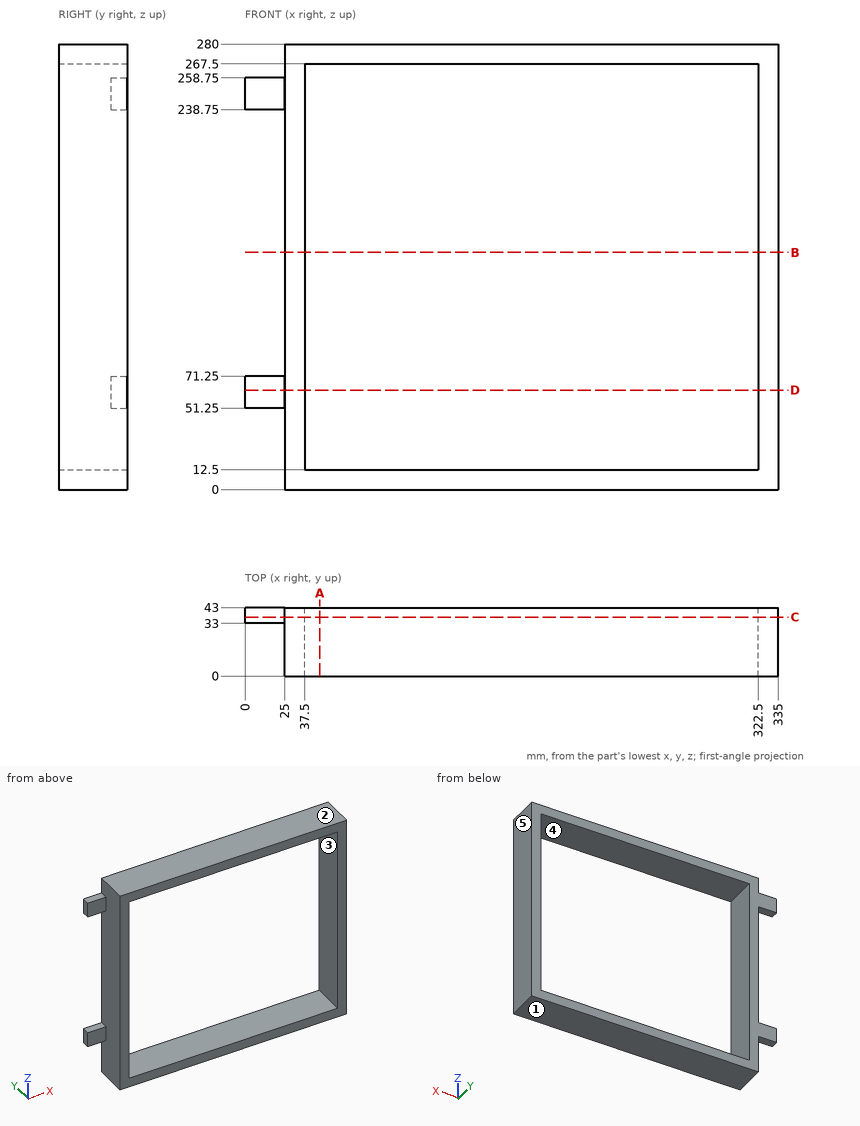
Here's the drawing with two shaded views (mm, measured from the low corner). I have some questions. A direction names the side the tool comes from. Round coordinates to 2 decimals unless told otherwise and drop trailing zeros. Order: outer loops, then holes, each group sorted by start corner. A loop starts at its lowest first (then second) coordinate and runs counter-clockwise, first axis right, second up. Notation, with made-up numbers: M 55,55.25 L 100,55.25 A14 ccw 100,76.25 Z; hole C 1.25,84.5 d3. An arc over 180 degrees is marked long. Answer in a Markdown table with one row per item.
Item 1: Imagine slicing it at C-C, the plane y = 37. Write out the boundary of the cut face in (x, z).
A:
| item | result |
|---|---|
| outline | M 0,51.25 L 25,51.25 L 25,0 L 335,0 L 335,280 L 25,280 L 25,258.75 L 0,258.75 L 0,238.75 L 25,238.75 L 25,71.25 L 0,71.25 Z; hole M 37.5,12.5 L 322.5,12.5 L 322.5,267.5 L 37.5,267.5 Z |
Item 2: Imagine slicing it at A-A, the plane x = 47. Write out the boundary of the cut face in (y, z).
A:
| item | result |
|---|---|
| outline | M 0,0 L 43,0 L 43,12.5 L 0,12.5 Z; M 0,267.5 L 43,267.5 L 43,280 L 0,280 Z |
Item 3: If I drill on L1, parallel to Z at x = 251.5, y = 13; L2, parallel to X at y = 40, z = 257; L3, parallel to X at y = 13, z = 101, over which ranges is the centre line in solid material (lowest first)? Write a range as from..to.
A:
| item | result |
|---|---|
| L1 | z = 0..12.5, 267.5..280 |
| L2 | x = 0..37.5, 322.5..335 |
| L3 | x = 25..37.5, 322.5..335 |
Item 4: Imagine slicing it at D-D, the plane z = 62.5. Write out the boundary of the cut face in (x, y), and give its area (4 significant figures).
A:
| item | result |
|---|---|
| outline | M 0,33 L 25,33 L 25,0 L 37.5,0 L 37.5,43 L 0,43 Z; M 322.5,0 L 335,0 L 335,43 L 322.5,43 Z |
| area | 1,325 mm2 |
Item 5: I'm going to push flat-ended pins straight in: pin 1 (8 mm diameter, centred on x = 15.5, y = 37, fed in from -Z); pin 2 (5 mm diameter, centred on x = 7, y = 39, fed in from +Z); pin 3 (21.5 mm diameter, centred on y = 29.5, z = 101.5, fed in from -X). Where does each tip first touch, or does it pass through?
A:
| item | result |
|---|---|
| pin 1 | stops at z = 51.25 |
| pin 2 | stops at z = 258.75 |
| pin 3 | stops at x = 25 |
Item 6: Imagine slicing it at B-B, the plane z = 149. Write out the boundary of the cut face in (x, y).
A:
| item | result |
|---|---|
| outline | M 25,0 L 37.5,0 L 37.5,43 L 25,43 Z; M 322.5,0 L 335,0 L 335,43 L 322.5,43 Z |
Item 7: Thinking about a two-plate mould opening in Z: for the marked faces 1, 2 and 3, which applies, +Z half, -Z half, draft (parallel to the pull), parting line (faces both ways), or undercut?
A:
| item | result |
|---|---|
| face 1 | -Z half |
| face 2 | +Z half |
| face 3 | undercut |
Item 8: For the marked faces 4 and 5, which set-ups out of +Z, -Z, +X, -X, +Y, -Y let a thin tool reach every point of the face, with its end or its side?
A:
| item | result |
|---|---|
| face 4 | +Y, -Y |
| face 5 | +Z, -Z, +X, +Y, -Y |
